Input: part model. Units: mm. Frame: model coordinates. A direction names the side the tool comes from. Round coordinates to 2 decimals unless told otherwise and drop trailing zeros. Loops run counter-clockwise (first coordinate to the right, second up) from the corner with the lowest first, then second, coordinate; pieces in that order, holes last. Notation, with made-up numbers: M -18.75,0.25 L 5.25,0.25 A31 cw 5.25,34.25 Z; hole C 8,35 d7. An arc over 180 degrees is marked long. Use one line per item in the form item = value. Start each with the question number.
Q1. Section query A-A, the plane z = 19.5. Output: boundary loops of the cut face in (x, y), and give its area (3 significant figures).
Q2. Section query C-C, the plane y = -17.5. Output: boundary loops of the cut face in (x, z).
Q3. First-contact query: P1, Ø6.5, axis at y = -7.5, z = 11.5, coming from the -X side; P2, Ø4.5, axis at x = 19, z = 14, coming from the +Y side; P3, Ø3, axis at x = 19, z = 3, coming from the +Y side; P4, Ø8, axis at x = 21.5, y = 22.5, coming from the +Z side. Flat tips, straight axial feed; report the tip coordinate or a pass-through.
Q4. Section query D-D, the plane x = -7.5. Output: boundary loops of the cut face in (y, z), and give its area (3 significant figures).
Q5. Section query B-B, the plane x = 21. Output: boundary loops of the cut face in (y, z), and give its area (3 significant figures).
Q6. Mould query, pull axis Y, two halves, no side actions, for faces 1 (the flat face through (-2, -29, 0)), 2 (the cylindrical face through (10.6, 39.32, 12.88)), 3 (the flat face through (20, 29.768, 14)). Classes: pulls with the +Y half, pulls with the -Y half, needs draft (parallel to the pull), parting line crosses it, or undercut.
Q7. Access query for faces 4 (the flat face through (-44.105, 0, 2)), 5 (the cylindrical face through (35.06, 26.71, 14.45)), 6 (the cylindrical face through (33.45, -26.81, 12.88)), 7 (the flat face through (37.957, -1, 14)), 8 (the cylindrical face through (-15.469, 40.107, 12.522)). Directions: +Z, -Z, +X, -X, +Y, -Y. A direction counts if a zero-diameter tool reaches every point of the face in a straight line with its end or side. Return the directions, or none.
Q8. Ray query, line 1 along X through (y, z) = (8, 4.5); line 2 along Y through (x, z) = (1, 24); line 3 along Y through (x, z) = (24, 8.5). Return the intervals inside material, ascending.
```python
from build123d import *

# Parameters (mm, degrees)
F2_DEPTH  = 25.4
F4_DEPTH  = 25.4
F5_DEPTH  = 3.81
F6_DEPTH  = 25.4
F8_DEPTH  = 25.4
F10_DEPTH = 25.4


with BuildPart() as f2:
    # F1 (on Top) → F2 (new body)
    with BuildSketch(Plane.XY):
        with BuildLine():
            Line((27.797497, 29.7675), (-31.882503, 29.7675))
            ThreePointArc((-31.882503, 29.7675), (-39.066708, 26.791705), (-42.042503, 19.6075))
            Line((-42.042503, 19.6075), (-42.042503, -21.0725))
            ThreePointArc((-42.042503, -21.0725), (-39.066708, -28.256705), (-31.882503, -31.2325))
            Line((-31.882503, -31.2325), (27.797497, -31.2325))
            ThreePointArc((27.797497, -31.2325), (34.981702, -28.256705), (37.957497, -21.0725))
            Line((37.957497, -21.0725), (37.957497, 19.6075))
            ThreePointArc((37.957497, 19.6075), (34.981702, 26.791705), (27.797497, 29.7675))
        make_face()
    extrude(amount=F2_DEPTH)

    # F3 (on face) → F4 (cut)
    with BuildSketch(Plane.XY.offset(25.4)):
        with BuildLine():
            Line((29.901702, 26.791705), (-33.986708, 26.791705))
            ThreePointArc((-33.986708, 26.791705), (-37.57881, 25.303808), (-39.066708, 21.711705))
            Line((-39.066708, 21.711705), (-39.066708, -23.176705))
            ThreePointArc((-39.066708, -23.176705), (-37.57881, -26.768807), (-33.986708, -28.256705))
            Line((-33.986708, -28.256705), (29.901702, -28.256705))
            ThreePointArc((29.901702, -28.256705), (33.493804, -26.768807), (34.981702, -23.176705))
            Line((34.981702, -23.176705), (34.981702, 21.711705))
            ThreePointArc((34.981702, 21.711705), (33.493804, 25.303808), (29.901702, 26.791705))
        make_face()
    extrude(amount=-F4_DEPTH, mode=Mode.SUBTRACT)

    # F0 (on Top) → F5 (join)
    with BuildSketch(Plane.XY):
        with BuildLine():
            Line((29.734908, 31.703549), (-33.945092, 31.703549))
            ThreePointArc((-33.945092, 31.703549), (-41.129297, 28.727754), (-44.105092, 21.543549))
            Line((-44.105092, 21.543549), (-44.105092, -23.136451))
            ThreePointArc((-44.105092, -23.136451), (-41.129297, -30.320656), (-33.945092, -33.296451))
            Line((-33.945092, -33.296451), (29.734908, -33.296451))
            ThreePointArc((29.734908, -33.296451), (36.919113, -30.320656), (39.894908, -23.136451))
            Line((39.894908, -23.136451), (39.894908, 21.543549))
            ThreePointArc((39.894908, 21.543549), (36.919113, 28.727754), (29.734908, 31.703549))
        make_face()
    extrude(amount=F5_DEPTH)

    # F5_face (on face) → F6 (cut)
    with BuildSketch(Plane(origin=(-2.042503, -0.7325, 3.81), x_dir=(1, 0, 0), z_dir=(0, 0, 1))):
        with BuildLine():
            Line((31.944205, 27.524205), (-31.944205, 27.524205))
            ThreePointArc((-31.944205, 27.524205), (-35.536307, 26.036307), (-37.024205, 22.444205))
            Line((-37.024205, 22.444205), (-37.024205, -22.444205))
            ThreePointArc((-37.024205, -22.444205), (-35.536307, -26.036307), (-31.944205, -27.524205))
            Line((-31.944205, -27.524205), (31.944205, -27.524205))
            ThreePointArc((31.944205, -27.524205), (35.536307, -26.036307), (37.024205, -22.444205))
            Line((37.024205, -22.444205), (37.024205, 22.444205))
            ThreePointArc((37.024205, 22.444205), (35.536307, 26.036307), (31.944205, 27.524205))
        make_face()
    extrude(amount=-F6_DEPTH, mode=Mode.SUBTRACT)

    # F7 (on Top) → F8 (join)
    with BuildSketch(Plane.XY):
        with BuildLine():
            Line((-16.826013, 36.880544), (-16.826013, 26.793541))
            Line((-16.826013, 26.793541), (12.303987, 26.793541))
            Line((12.303987, 26.793541), (12.303987, 36.880544))
            ThreePointArc((12.303987, 36.880544), (10.98216, 40.071715), (7.790989, 41.393541))
            Line((7.790989, 41.393541), (-12.313015, 41.393541))
            ThreePointArc((-12.313015, 41.393541), (-15.504187, 40.071715), (-16.826013, 36.880544))
        make_face()
    extrude(amount=F8_DEPTH)

    # F9 (on face) → F10 (cut)
    with BuildSketch(Plane.XY.offset(25.4)):
        with BuildLine():
            Line((8.805542, 40.071715), (-12.990056, 40.071715))
            ThreePointArc((-12.990056, 40.071715), (-14.767815, 39.335343), (-15.504187, 37.557585))
            Line((-15.504187, 37.557585), (-15.504187, 26.791705))
            Line((-15.504187, 26.791705), (11.320142, 26.791705))
            Line((11.320142, 26.791705), (11.320142, 37.557115))
            ThreePointArc((11.320142, 37.557115), (10.583633, 39.335206), (8.805542, 40.071715))
        make_face()
    extrude(amount=-F10_DEPTH, mode=Mode.SUBTRACT)


solid = f2.part
```
Results found:
q1.outline = M -42.04,-21.07 A10.16 ccw -31.88,-31.23 L 27.8,-31.23 A10.16 ccw 37.96,-21.07 L 37.96,19.61 A10.16 ccw 27.8,29.77 L 12.3,29.77 L 12.3,36.88 A4.51 ccw 7.79,41.39 L -12.31,41.39 A4.51 ccw -16.83,36.88 L -16.83,29.77 L -31.88,29.77 A10.16 ccw -42.04,19.61 Z; hole M -39.07,-23.18 A5.08 ccw -33.99,-28.26 L 29.9,-28.26 A5.08 ccw 34.98,-23.18 L 34.98,21.71 A5.08 ccw 29.9,26.79 L 11.32,26.79 L 11.32,37.56 A2.51 ccw 8.81,40.07 L -12.99,40.07 A2.51 ccw -15.5,37.56 L -15.5,26.79 L -33.99,26.79 A5.08 ccw -39.07,21.71 Z
q1.area = 714 mm²
q2.outline = M -44.11,0 L -39.07,0 L -39.07,25.4 L -42.04,25.4 L -42.04,3.81 L -44.11,3.81 Z; M 34.98,0 L 39.89,0 L 39.89,3.81 L 37.96,3.81 L 37.96,25.4 L 34.98,25.4 Z
q3.P1 = -42.04
q3.P2 = 29.77
q3.P3 = 31.7
q3.P4 = through
q4.outline = M -33.3,0 L -28.26,0 L -28.26,25.4 L -31.23,25.4 L -31.23,3.81 L -33.3,3.81 Z; M 40.07,0 L 41.39,0 L 41.39,25.4 L 40.07,25.4 Z
q4.area = 117 mm²
q5.outline = M -33.3,0 L -28.26,0 L -28.26,25.4 L -31.23,25.4 L -31.23,3.81 L -33.3,3.81 Z; M 26.79,0 L 31.7,0 L 31.7,3.81 L 29.77,3.81 L 29.77,25.4 L 26.79,25.4 Z
q5.area = 166 mm²
q6.face_1 = needs draft
q6.face_2 = undercut
q6.face_3 = pulls with the +Y half
q7.face_4 = +Z, -Z, -X, +Y, -Y
q7.face_5 = +Z, +X, +Y
q7.face_6 = +Z, -Z
q7.face_7 = +Z, +X, +Y, -Y
q7.face_8 = +Z, -Z, -X, +Y
q8.line_1 = -42.04 to -39.07, 34.98 to 37.96
q8.line_2 = -31.23 to -28.26, 40.07 to 41.39
q8.line_3 = -31.23 to -28.26, 26.79 to 29.77
